Design review of the part built by this model. Coordinates are the model's own, in mm. A direction names the side the tool comes from. Coordinates: 2 decimals unless noted, no trailing zeros. Write each loop counter-clockwise with the first axis right and the second up, starting at its lowest first coordinate (ties: lowest second). Pieces come first, ordered by that corner, then holes. Notation, with made-up numbers: (-38.5, 18) - (13.5, 18) arc R5 cw to (13.5, 23) - close; hole circle Ø5 at (88.25, 51.5). An arc over 180 degrees is marked (long way). Use a Markdown table: item, result.
from build123d import *

# Parameters (mm, degrees)
SKETCH1_R           = 4
SKETCH1_R_2         = 5
SKETCH1_R_3         = 1.75
BOSS_EXTRUDE1_DEPTH = 6
CHAMFER1_SIZE       = 6
CUT_EXTRUDE2_DEPTH  = 10
SKETCH4_W           = 3
SKETCH4_H           = 5.7
CUT_EXTRUDE3_DEPTH  = 38.107950631
CUT_EXTRUDE4_START  = -6
SKETCH2_R           = 8.075
CUT_EXTRUDE4_DEPTH  = 5
SKETCH5_R           = 1.75
CUT_EXTRUDE5_DEPTH  = 5


with BuildPart() as part:
    # Sketch1 → Boss-Extrude1 (new body)
    with BuildSketch(Plane.XY):
        Polygon((-21, -30), (21, -30), (21, 30), (-21, 30), (-21, -8), align=None)
        with Locations((-10, -23)):
            Circle(SKETCH1_R, mode=Mode.SUBTRACT)
        with Locations((-10, -8)):
            Circle(SKETCH1_R_2, mode=Mode.SUBTRACT)
        with Locations(Location((10, -8, 0), (0, 0, 180))):
            Circle(SKETCH1_R_2, mode=Mode.SUBTRACT)
        with Locations(Location((10, -23, 0), (0, 0, 180))):
            Circle(SKETCH1_R, mode=Mode.SUBTRACT)
        with Locations((16, 27)):
            Circle(SKETCH1_R_3, mode=Mode.SUBTRACT)
        with Locations(Location((-16, 27, 0), (0, 0, 180))):
            Circle(SKETCH1_R_3, mode=Mode.SUBTRACT)
    extrude(amount=BOSS_EXTRUDE1_DEPTH)

    # Chamfer1
    # the kernel refuses this chamfer: 6 mm, written as the material it takes off along each edge
    with BuildSketch(Plane(origin=(-36.430097928, -30, 0), x_dir=(0, -0.027495876610586202, 0.9996219169112968), z_dir=(1, 0, 0))) as chamfer1_piece_1:
        Polygon((CHAMFER1_SIZE * 0.999621916911, -CHAMFER1_SIZE * 0.0274958766106), (-CHAMFER1_SIZE * 0.0274958766106, -CHAMFER1_SIZE * 0.999621916911), (0, 0), align=None)
    extrude(amount=72.860195856, mode=Mode.SUBTRACT)

    # Sketch3 → Cut-Extrude2 (cut)
    with BuildSketch(Plane(origin=(0, 0, 0), x_dir=(-1, 0, 0), z_dir=(0, 0, -1))):
        Polygon((9.6, 14), (9.611608629, 1.1), (21, 1.1), (21, 14), align=None)
    extrude(amount=-CUT_EXTRUDE2_DEPTH, mode=Mode.SUBTRACT)

    # Sketch4 → Cut-Extrude3 (cut, through all)
    with BuildSketch(Plane(origin=(0, 0, 0), x_dir=(-1, 0, 0), z_dir=(0, 0, -1))):
        with Locations((-18.5, -16)):
            Rectangle(SKETCH4_W, SKETCH4_H)
        with Locations((18.5, -16)):
            Rectangle(SKETCH4_W, SKETCH4_H)
        with Locations((-18.5, 19)):
            Rectangle(SKETCH4_W, SKETCH4_H)
        with Locations((18.5, 19)):
            Rectangle(SKETCH4_W, SKETCH4_H)
    extrude(amount=-CUT_EXTRUDE3_DEPTH, mode=Mode.SUBTRACT)

    # Sketch2 → Cut-Extrude4 (cut)
    with BuildSketch(Plane.XY.offset(6).offset(CUT_EXTRUDE4_START)):
        with Locations((-10, -8)):
            Circle(SKETCH2_R)
        with Locations(Location((10, -8, 0), (0, 0, 180))):
            Circle(SKETCH2_R)
    extrude(amount=CUT_EXTRUDE4_DEPTH, mode=Mode.SUBTRACT)

    # Sketch5 → Cut-Extrude5 (cut)
    with BuildSketch(Plane(origin=(21, 0, 0), x_dir=(0, 0, -1), z_dir=(1, 0, 0))):
        with Locations(Location((-3, -16, 0), (0, 0, 90))):
            Circle(SKETCH5_R)
        with Locations(Location((-3, 19, 0), (0, 0, 90))):
            Circle(SKETCH5_R)
    cut_extrude5 = extrude(amount=-CUT_EXTRUDE5_DEPTH, mode=Mode.SUBTRACT)

    # Mirror1: Cut-Extrude5 across plane
    add(cut_extrude5.mirror(Plane(origin=(0, 0, 0), x_dir=(0, 0, 1), z_dir=(1, 0, 0))), mode=Mode.SUBTRACT)


solid = part.part
(1) Take a section at B-B on x = 10. Write out the cut boundary in (y, z) (3 decimals).
Determined:
| item | result |
|---|---|
| outline | (-30, 6) - (-27, 3) - (-27, 6) - close; (-19, 0) - (-16.075, 0) - (-16.075, 5) - (-13, 5) - (-13, 6) - (-19, 6) - close; (-3, 5) - (0.075, 5) - (0.075, 0) - (30, 0) - (30, 6) - (-3, 6) - close |
(2) Take a section at D-D on x = -11. Write out the cut boundary in (y, z), and give its area (3 significant figures).
Determined:
| item | result |
|---|---|
| outline | (-30, 6) - (-26.87, 2.87) - (-26.87, 6) - close; (-19.13, 0) - (-16.01, 0) - (-16.01, 5) - (-12.9, 5) - (-12.9, 6) - (-19.13, 6) - close; (-3.1, 5) - (0.01, 5) - (0.01, 0) - (1.1, 0) - (1.1, 6) - (-3.1, 6) - close; (14, 0) - (30, 0) - (30, 6) - (14, 6) - close |
| area | 132 mm2 |
(3) Machinability: for faces 1 (the cylindrical face through (15.95, -13.46, 2.46)), 2 (the flat face through (0, 30, 3)), 3 (the flat face through (-18, 16.15, 3)), 4 (the cylindrical face through (20.507, -14.383, 2.33)), 5 (the cylindrical face through (-16.51, 17.25, 3.08)), which of the approach directions +Z, -Z, +X, -X, +Y, -Y give a long, thin tool a straight path to every point of the face, cutting with its end or side? Answer none if there is none.
Determined:
| item | result |
|---|---|
| face 1 | -Z |
| face 2 | +Z, -Z, +X, -X, +Y |
| face 3 | +Z, -Z |
| face 4 | +X |
| face 5 | -X |
(4) For pin 1 (10.5 mm diameter, centred on x = -10, y = -23, fed in from -Z); pin 2 (3 mm diameter, centred on y = 19, z = 3, fed in from +X); pin 3 (3 mm diameter, centred on y = -16, z = 3, fed in from -X); pin 4 (0.9 mm diameter, centred on x = 19, z = 3.5, fed in from -Y), all flat-tipped, find the tip position at first contact; note any pin that passes through.
Determined:
| item | result |
|---|---|
| pin 1 | z = 0 |
| pin 2 | x = 16 |
| pin 3 | x = -16 |
| pin 4 | y = -27.95 |
(5) Take a section at C-C on y = 19. Write out the cut boundary in (x, z).
Determined:
| item | result |
|---|---|
| outline | (-21, 0) - (-20, 0) - (-20, 1.25) - (-21, 1.25) - close; (-21, 4.75) - (-20, 4.75) - (-20, 6) - (-21, 6) - close; (-17, 0) - (17, 0) - (17, 1.25) - (16, 1.25) - (16, 4.75) - (17, 4.75) - (17, 6) - (-17, 6) - (-17, 4.75) - (-16, 4.75) - (-16, 1.25) - (-17, 1.25) - close; (20, 0) - (21, 0) - (21, 1.25) - (20, 1.25) - close; (20, 4.75) - (21, 4.75) - (21, 6) - (20, 6) - close |
(6) Take a section at A-A on y = 27. Write out the cut boundary in (x, z).
Determined:
| item | result |
|---|---|
| outline | (-21, 0) - (-17.75, 0) - (-17.75, 6) - (-21, 6) - close; (-14.25, 0) - (14.25, 0) - (14.25, 6) - (-14.25, 6) - close; (17.75, 0) - (21, 0) - (21, 6) - (17.75, 6) - close |
(7) For L1, parallel to X at y = -23, z = 4; L2, parallel to Y at x = -20.5, z = 3; L3, parallel to X at y = -11, z = 1.75, list the stretches that pass through material, from the lowest coordinate up. Write a range as from..to.
Determined:
| item | result |
|---|---|
| L1 | -21..-14, -6..6, 14..21 |
| L2 | -27..-17.75, -14.25..1.1, 14..17.25, 20.75..30 |
| L3 | -21..-17.5, -2.5..2.5, 17.5..21 |
(8) Draft analysis for pull direction X (two halves, no side actions). For faces 6 (the flat face through (-20, 17.7, 1.6)), 7 (the flat face through (-15, 14, 3)), 8 (the flat face through (16, 19, 3)), 9 (the flat face through (-18, -18.85, 3)), state which applies: +X half, -X half, draft (parallel to the pull), parting line (faces both ways), or undercut.
Determined:
| item | result |
|---|---|
| face 6 | undercut |
| face 7 | draft |
| face 8 | +X half |
| face 9 | undercut |
